```python
from build123d import *

# Parameters (mm, degrees)
SKETCH1_W           = 23
SKETCH1_H           = 20
BOSS_EXTRUDE1_DEPTH = 17
SKETCH2_R           = 7.5
SKETCH2_R_2         = 1
BOSS_EXTRUDE2_DEPTH = 3
SKETCH3_W           = 3
SKETCH3_H           = 10
CUT_EXTRUDE1_DEPTH  = 8
SKETCH4_R           = 1
CUT_EXTRUDE2_DEPTH  = 33.634337744


with BuildPart() as part:
    # Sketch1 → Boss-Extrude1 (new, symmetric)
    with BuildSketch(Plane(origin=(0, 0, 0), x_dir=(1, 0, 0), z_dir=(0, 1, 0))):
        Rectangle(SKETCH1_W, SKETCH1_H)
    extrude(amount=BOSS_EXTRUDE1_DEPTH, both=True)

    # Sketch2 → Boss-Extrude2 (add)
    with BuildSketch(Plane(origin=(11.5, 0, 0), x_dir=(0, 0, -1), z_dir=(1, 0, 0))):
        with Locations((0, 7)):
            Circle(SKETCH2_R)
        with Locations((0, 13)):
            Circle(SKETCH2_R_2, mode=Mode.SUBTRACT)
        with Locations((6, 7)):
            Circle(SKETCH2_R_2, mode=Mode.SUBTRACT)
        with Locations((0, 1)):
            Circle(SKETCH2_R_2, mode=Mode.SUBTRACT)
        with Locations((-6, 7)):
            Circle(SKETCH2_R_2, mode=Mode.SUBTRACT)
    boss_extrude2 = extrude(amount=BOSS_EXTRUDE2_DEPTH)

    # Mirror1: Boss-Extrude2 across plane
    add(boss_extrude2.mirror(Plane(origin=(0, 0, 0), x_dir=(0, 0, 1), z_dir=(1, 0, 0))))

    # Sketch3 → Cut-Extrude1 (cut)
    with BuildSketch(Plane(origin=(11.5, 0, 0), x_dir=(0, 0, -1), z_dir=(1, 0, 0))):
        with Locations((-8.5, -5)):
            Rectangle(SKETCH3_W, SKETCH3_H)
        with Locations((8.5, -5)):
            Rectangle(SKETCH3_W, SKETCH3_H)
    cut_extrude1 = extrude(amount=-CUT_EXTRUDE1_DEPTH, mode=Mode.SUBTRACT)

    # Mirror2: Cut-Extrude1 across plane
    add(cut_extrude1.mirror(Plane(origin=(0, 0, 0), x_dir=(0, 0, 1), z_dir=(1, 0, 0))), mode=Mode.SUBTRACT)

    # Sketch4 → Cut-Extrude2 (cut, through all)
    with BuildSketch(Plane(origin=(11.5, 0, 0), x_dir=(0, 0, -1), z_dir=(1, 0, 0))):
        with Locations((-8, 15)):
            Circle(SKETCH4_R)
        with Locations((8, 15)):
            Circle(SKETCH4_R)
        with Locations((-8, -15)):
            Circle(SKETCH4_R)
        with Locations((8, -15)):
            Circle(SKETCH4_R)
    extrude(amount=-CUT_EXTRUDE2_DEPTH, mode=Mode.SUBTRACT)


solid = part.part
```
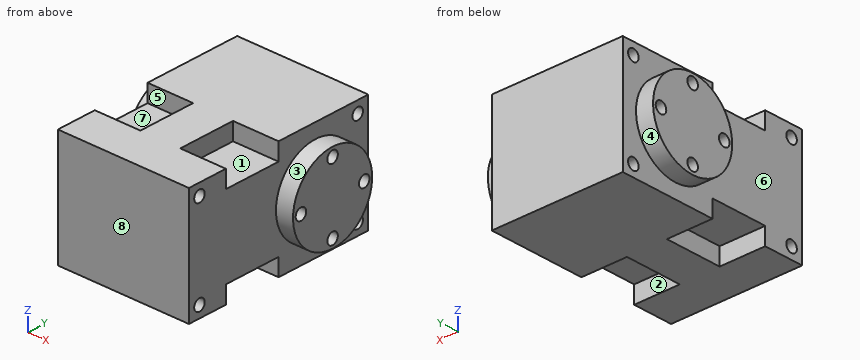
Read the model definition and answer for the solid it produces. Units are mm, in the model's axes. Face numbers are marked on the shaded views. A direction names the side the tool comes from. Give positions to 0.01 mm unless a question says otherwise; leave off trailing zeros. Write each loop counter-clockwise with the first axis right and the second up, starting at its lowest first coordinate (ties: lowest second). Pieces come first, ordered by that corner, then holes. Notation, with made-up numbers: M -20,-5.75 L -7,-5.75 A11 cw -7,1.25 Z; hole C -12,31 d4. An arc over 180 degrees is marked long. Put each result on its own line as item: value. Start each with the question number.
1. Consider line 1 along Y through (x, z) = (-1.25, 8); line 2 along Y through (x, z) = (-1.5, 8.75); line 3 along X through (y, z) = (-8, 4.5). Determine where each line is inside the solid, lowest interval first.
2. For a pull along Y with two mould halves and no side action, classify the marked faces 6, 7 and 8 as released by +Y, released by -Y, zero draft, split by the parting line, or undercut.
3. Each of these flat-tipped pins is pushed along its axis until it touches: pin 1 Ø3.5 at (y, z) = (-4, -8.5) entering from -X; pin 2 Ø2 at (x, y) = (10, -2.5) entering from -Z; pin 3 Ø5 at (y, z) = (-7, -0.5) entering from +X. Where does it stop, or does it pass through?
4. The part is cut by section C-C, the plane y = 1. Give the vertices of the cut face in (x, z).
5. Which of the six approach directions +Z, -Z, +X, -X, +Y, -Y give full straight-line access (tool end or side, diameter ignored) to the marked faces 1, 2, 3, 4 and 5?
6. The part is cut by section A-A, the plane y = 15. Give the vertices of the cut face in (x, z).
7. The part is cut by section D-D, the plane z = 6. Give the vertices of the cut face in (x, y), and give its area (3 significant figures).
8. The part is cut by section B-B, the plane z = -8. Give the vertices of the cut face in (x, y).
Final values:
1. line 1: y = -17 to -16, -14 to 14, 16 to 17
1. line 2: y = -17 to -15.66, -14.34 to 14.34, 15.66 to 17
1. line 3: x = -11.5 to 11.5
2. face 6: zero draft
2. face 7: undercut
2. face 8: released by -Y
3. pin 1: stops at x = -11.5
3. pin 2: stops at z = -7
3. pin 3: stops at x = 11.5
4. outline: M -14.5,-4.5 L -11.5,-4.5 L -11.5,-10 L 11.5,-10 L 11.5,-4.5 L 14.5,-4.5 L 14.5,-1 L 11.5,-1 L 11.5,1 L 14.5,1 L 14.5,4.5 L 11.5,4.5 L 11.5,10 L -11.5,10 L -11.5,4.5 L -14.5,4.5 L -14.5,1 L -11.5,1 L -11.5,-1 L -14.5,-1 Z
5. face 1: +Z, +X
5. face 2: -Z, +X
5. face 3: +X
5. face 4: -X
5. face 5: +Z, -X
6. outline: M -11.5,-10 L 11.5,-10 L 11.5,-9 L -11.5,-9 Z; M -11.5,-7 L 11.5,-7 L 11.5,7 L -11.5,7 Z; M -11.5,9 L 11.5,9 L 11.5,10 L -11.5,10 Z
7. outline: M -14.5,2.5 L -11.5,2.5 L -11.5,-17 L 11.5,-17 L 11.5,2.5 L 14.5,2.5 L 14.5,6 L 11.5,6 L 11.5,8 L 14.5,8 L 14.5,11.5 L 11.5,11.5 L 11.5,17 L -11.5,17 L -11.5,11.5 L -14.5,11.5 L -14.5,8 L -11.5,8 L -11.5,6 L -14.5,6 Z
7. area: 824 mm²
8. outline: M -11.5,-17 L 11.5,-17 L 11.5,-16 L -11.5,-16 Z; M -11.5,-14 L 11.5,-14 L 11.5,-10 L 3.5,-10 L 3.5,0 L 11.5,0 L 11.5,14 L -11.5,14 L -11.5,0 L -3.5,0 L -3.5,-10 L -11.5,-10 Z; M -11.5,16 L 11.5,16 L 11.5,17 L -11.5,17 Z
